Can you work these out from the drawing? Everything is in mm from the part's minimum corner. A direction names the side the tool comes from. Coordinates: 2 decimals unless noted, no trailing zeros. Order: outer loops, then holes, each group sorted by start corner. A loop starts at its lowest first (then second) coordinate and runs counter-clockwise, first axis right, second up. Notation, with made-up numbers: (-24.5, -3) -> (25.5, -3) arc R19 ccw to (25.5, 26) -> close; hole circle Ø11 at (49.25, 84). An arc over 180 degrees is marked (long way). Use a Markdown table: item, result. Add a question column.
1) If we section it at C-C (z = 13.5): Write out the boundary of the cut face in (x, y), plus the area to 3 significant figures.
2) Will these pins go through, and if not, where does the flat tip stop? pin 1 Ø16 at (x, z) = (12, 29.39) entering from -Y; pin 2 Ø6.5 at (x, z) = (33.5, 34) entering from +Y; pin 3 Ø6 at (x, y) = (23.98, 19.33) entering from +Z; pin 4 Ø1 at (x, y) = (25.5, 1) entering from -Z.
3) If we section it at D-D (z = 26.5): Write out the boundary of the cut face in (x, y), plus the area to 3 significant figures.
4) Which directions (+Z, -Z, +X, -X, +Y, -Y) give clear straight access to the entire face, cutting with the end or side of a thin tool? Please do the marked faces 5, 6, 7 and 8.
5) If we section it at A-A (x = 36): Write out the boundary of the cut face in (y, z).
6) Thinking about a two-plate mould opening in X: for the marked faces 1, 2, 3 and 4, which applies, +X half, -X half, draft (parallel to the pull), parting line (faces both ways), or undercut?
7) If we section it at B-B (y = 18.5): Write out the boundary of the cut face in (x, z).
8) If I drill on L1, parallel to X at y = 14, z = 10.5; L2, parallel to Y at x = 23, z = 24, over which ranges is the centre line in solid material (lowest first)? Write a range as [from, to].
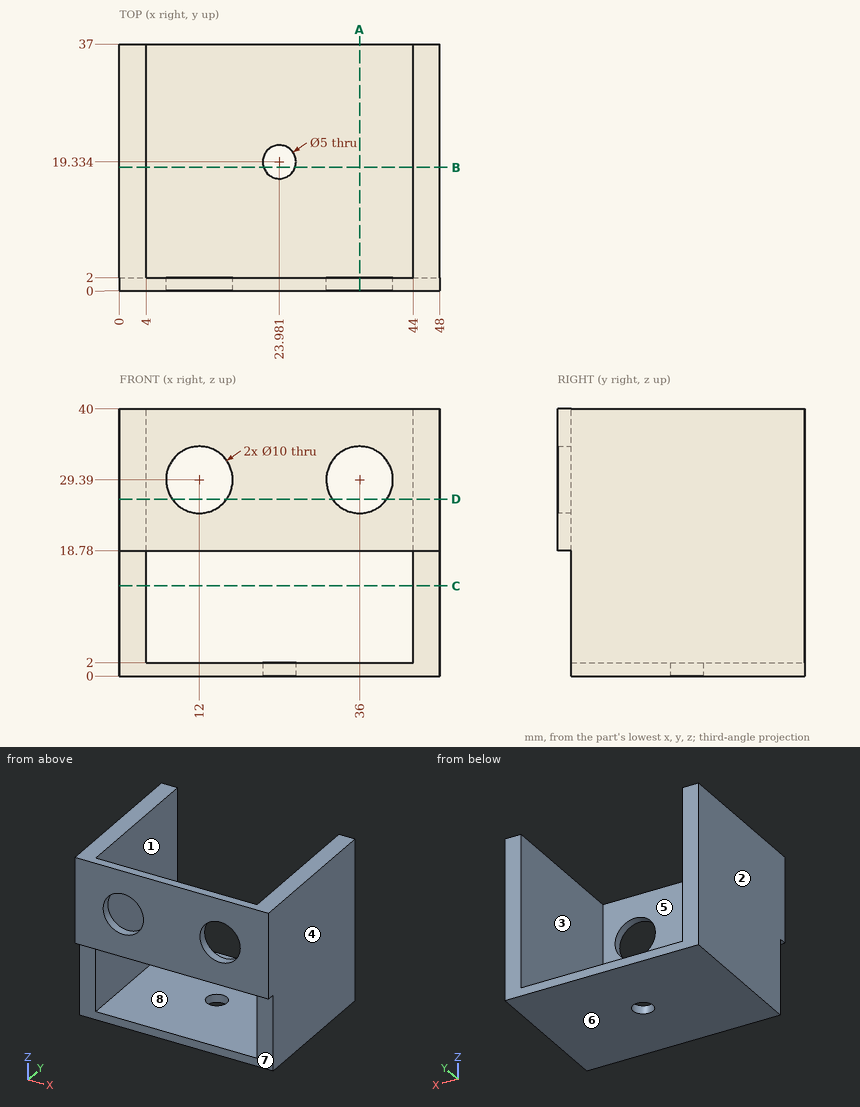
Answer sheet:
| question | item | result |
|---|---|---|
| 1 | outline | (0, 2) -> (4, 2) -> (4, 37) -> (0, 37) -> close; (44, 2) -> (48, 2) -> (48, 37) -> (44, 37) -> close |
| 1 | area | 280 mm2 |
| 2 | pin 1 | y = 0 |
| 2 | pin 2 | y = 2 |
| 2 | pin 3 | z = 2 |
| 2 | pin 4 | z = 18.78 |
| 3 | outline | (0, 0) -> (7.92, 0) -> (7.92, 2) -> (4, 2) -> (4, 37) -> (0, 37) -> close; (16.08, 0) -> (31.92, 0) -> (31.92, 2) -> (16.08, 2) -> close; (40.08, 0) -> (48, 0) -> (48, 37) -> (44, 37) -> (44, 2) -> (40.08, 2) -> close |
| 3 | area | 343 mm2 |
| 4 | face 5 | +Z, +Y |
| 4 | face 6 | -Z, +X, -X, +Y, -Y |
| 4 | face 7 | -Z, +X, -X, -Y |
| 4 | face 8 | +Z, +Y, -Y |
| 5 | outline | (0, 18.78) -> (2, 18.78) -> (2, 24.39) -> (0, 24.39) -> close; (0, 34.39) -> (2, 34.39) -> (2, 40) -> (0, 40) -> close; (2, 0) -> (37, 0) -> (37, 2) -> (2, 2) -> close |
| 6 | face 1 | undercut |
| 6 | face 2 | -X half |
| 6 | face 3 | undercut |
| 6 | face 4 | +X half |
| 7 | outline | (0, 0) -> (21.62, 0) -> (21.62, 2) -> (4, 2) -> (4, 40) -> (0, 40) -> close; (26.34, 0) -> (48, 0) -> (48, 40) -> (44, 40) -> (44, 2) -> (26.34, 2) -> close |
| 8 | L1 | [0, 4], [44, 48] |
| 8 | L2 | [0, 2] |
